Build history of the part. All positions in model axes, mm. Face numbers are marked on the shaded views. Coordinates: 2 decimals unless noted, no trailing zeros. Return JSON: item names as keys, results as strings.
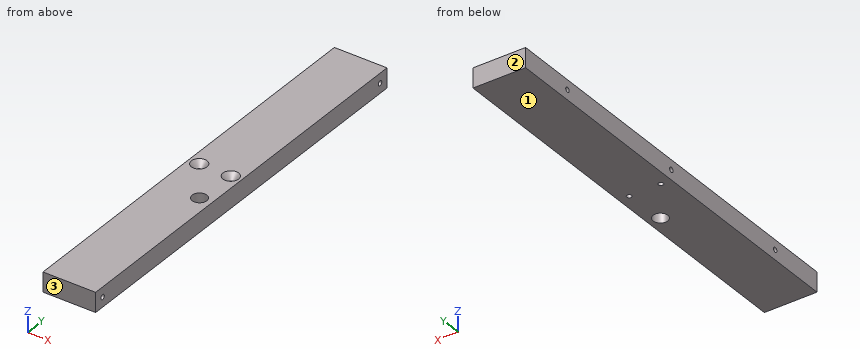
from build123d import *

# Parameters (mm, degrees)
SKETCH1_W                    = 34
SKETCH1_H                    = 265.399999988
BOSS_EXTRUDE1_DEPTH          = 12.7
F_3_8_0_375_DIAMETER_HOLE1_D = 9.525
HOLE1_D                      = 3.175
HOLE1_DEPTH                  = 31.75
HOLE1_CSINK_D                = 10.16
HOLE1_CSINK_ANGLE            = 82
HOLE1_TIP                    = 0.953866233
HOLE3_D                      = 3.175
HOLE3_DEPTH                  = 31.75
HOLE3_CSINK_D                = 10.16
HOLE3_CSINK_ANGLE            = 82
HOLE3_TIP                    = 0.953866233
HOLE4_D                      = 3.175
HOLE4_DEPTH                  = 31.75
HOLE4_CSINK_D                = 10.16
HOLE4_CSINK_ANGLE            = 82
HOLE4_TIP                    = 0.953866233


with BuildPart() as part:
    # Sketch1 → Boss-Extrude1 (new body)
    with BuildSketch(Plane.XY):
        with Locations((-23.08092085, 0)):
            Rectangle(SKETCH1_W, SKETCH1_H)
    extrude(amount=-BOSS_EXTRUDE1_DEPTH)

    # 3/8 (0.375) Diameter Hole1 (through all)
    with Locations(Plane.XY):
        with Locations((-14.118005489, -26.732654045)):
            Hole(F_3_8_0_375_DIAMETER_HOLE1_D / 2)

    # Hole1
    with Locations(Plane(origin=(12.91907915, 0, 155.024290059), x_dir=(0, -1, 0), z_dir=(1, 0, 0))):
        with Locations((126.349999994, 161.374290059), (146.083333327, 4.074290059), (172.166666661, 4.074290059), (126.349999994, 34.524290059), (126.349999994, 130.924290059), (-172.166666661, 4.074290059), (-146.083333327, 4.074290059), (-126.349999994, 34.524290059), (-126.349999994, 130.924290059), (-126.349999994, 161.374290059)):
            CounterSinkHole(HOLE1_D / 2, HOLE1_CSINK_D / 2, depth=HOLE1_DEPTH, counter_sink_angle=HOLE1_CSINK_ANGLE)
            with Locations((0, 0, -(HOLE1_DEPTH + HOLE1_TIP / 2))):  # 118° drill point
                Cone(0, HOLE1_D / 2, HOLE1_TIP, mode=Mode.SUBTRACT)

    # Hole3
    with Locations(Plane(origin=(-195.367659426, 0, 0), x_dir=(0, -1, 0), z_dir=(0, 0, 1))):
        with Locations((0, 162.086738577), (0, 182.486738577)):
            CounterSinkHole(HOLE3_D / 2, HOLE3_CSINK_D / 2, depth=HOLE3_DEPTH, counter_sink_angle=HOLE3_CSINK_ANGLE)
            with Locations((0, 0, -(HOLE3_DEPTH + HOLE3_TIP / 2))):  # 118° drill point
                Cone(0, HOLE3_D / 2, HOLE3_TIP, mode=Mode.SUBTRACT)

    # Hole4
    with Locations(Plane(origin=(-52.78092085, 0, 155.024290059), x_dir=(0, 1, 0), z_dir=(-1, 0, 0))):
        with Locations((-207.774999994, 333.02141023), (-207.774999994, 225.48903684), (-207.774999994, 137.424290059), (-172.166666661, 4.074290059), (-146.083333327, 4.074290059), (-94.599999994, 161.374290059), (0, 161.374290059), (94.599999994, 161.374290059), (146.083333327, 4.074290059), (172.166666661, 4.074290059), (207.774999994, 137.424290059), (207.774999994, 225.48903684), (207.774999994, 333.02141023), (166.795833328, 301.970350905), (40.979166666, 301.970350905), (-40.979166666, 301.970350905), (-166.795833328, 301.970350905), (0, 193.124290059), (0, 301.970350905), (0, 412.366411751), (-126.349999994, 106.824290059), (-126.349999994, 58.624290059), (126.349999994, 58.624290059), (126.349999994, 106.824290059)):
            CounterSinkHole(HOLE4_D / 2, HOLE4_CSINK_D / 2, depth=HOLE4_DEPTH, counter_sink_angle=HOLE4_CSINK_ANGLE)
            with Locations((0, 0, -(HOLE4_DEPTH + HOLE4_TIP / 2))):  # 118° drill point
                Cone(0, HOLE4_D / 2, HOLE4_TIP, mode=Mode.SUBTRACT)


solid = part.part
1. Drop flat-ended pins along their axis: pin 1 (8.5 mm diameter, centred on x = -14.12, y = -26.73, fed in from -Z) (1 decimal); pin 2 (4 mm diameter, centred on x = -12.88, y = 0, fed in from +Z); pin 3 (2.5 mm diameter, centred on y = -94.6, z = -6.35, fed in from -X). Give the stop position or say it passes through.
Check values:
{"pin 1": "through", "pin 2": "z = -3.54", "pin 3": "x = -20.83"}
2. Probe L1, parallel to Y at x = -10.5, z = -6; L2, parallel to Y at x = -10, z = -7; L3, parallel to Y at x = -15, z = -1.5. List the from-to ranges inside material, lowest first.
Check values:
{"L1": "-132.7 to -127.9, -124.8 to -29.83, -23.64 to 124.8, 127.9 to 132.7", "L2": "-132.7 to -127.8, -124.9 to -29.13, -24.34 to 124.9, 127.8 to 132.7", "L3": "-132.7 to -31.41, -22.05 to -3.13, 3.13 to 132.7"}
3. Mould opens along Y. For the marked faces 1, 2 and 3 say: pulls with the +Y half, pulls with the -Y half, needs draft (parallel to the pull), parting line crosses it, or undercut.
Check values:
{"face 1": "needs draft", "face 2": "pulls with the +Y half", "face 3": "pulls with the -Y half"}
